Here's how the part is built. I have some questions about the finished solid (model axes, mm). Face numbers are marked on the shaded views. Give positions to 0.01 mm unless a question says otherwise; leave off trailing zeros. Write each loop counter-clockwise with the first axis right and the second up, starting at its lowest first coordinate (ties: lowest second). Pieces come first, ordered by that corner, then holes. Notation, with made-up numbers: (1.25, -22) - (35.25, -22) arc R18 cw to (35.25, 8) - close; hole circle Ø2 at (57, 34.25). An arc over 180 degrees is marked (long way). Use one line per item in the form item = value. Start each with the question number.
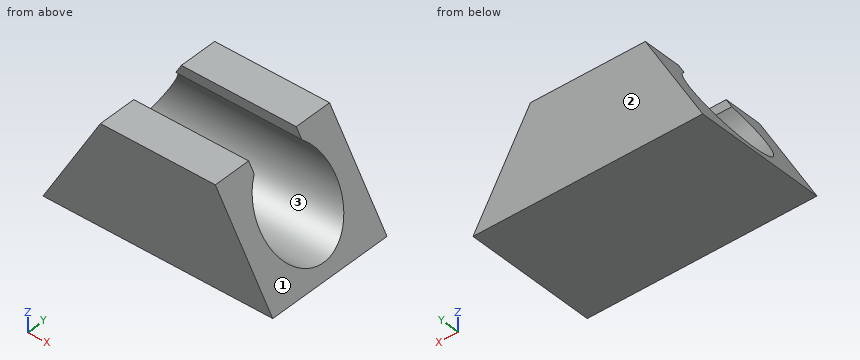
from build123d import *

# Parameters (mm, degrees)
SKETCH8_W           = 10.392304846
SKETCH8_H           = 6
BOSS_EXTRUDE3_DEPTH = 4.5
CUT_EXTRUDE5_DEPTH  = 11.392304845
CUT_EXTRUDE6_DEPTH  = 7


with BuildPart() as part:
    # Sketch8 → Boss-Extrude3 (new body)
    with BuildSketch(Plane.XY):
        Rectangle(SKETCH8_W, SKETCH8_H)
    extrude(amount=BOSS_EXTRUDE3_DEPTH)

    # Sketch9 → Cut-Extrude5 (cut, through all)
    with BuildSketch(Plane(origin=(5.196152423, 0, 0), x_dir=(0, 0, -1), z_dir=(1, 0, 0))):
        with BuildLine():
            Line((-4.0612495, 1.25), (-4.5, 1.25))
            Line((-4.5, 1.25), (-4.5, -1.25))
            Line((-4.5, -1.25), (-4.0612495, -1.25))
            ThreePointArc((-4.0612495, -1.25), (-0.5, 0), (-4.0612495, 1.25))
        make_face()
    extrude(amount=-CUT_EXTRUDE5_DEPTH, mode=Mode.SUBTRACT)

    # Sketch10 → Cut-Extrude6 (cut, through all)
    with BuildSketch(Plane.XZ.offset(3)):
        Polygon((5.196152423, 0), (2.598076211, 4.5), (5.196152423, 4.5), align=None)
        Polygon((-5.196152423, 4.5), (-5.196152423, 0), (-2.598076211, 4.5), align=None)
    extrude(amount=-CUT_EXTRUDE6_DEPTH, mode=Mode.SUBTRACT)


solid = part.part
1. We'd pull the mould along Y, two halves only. Please class the marked faces 1, 2 and 3: pulls with the +Y half, pulls with the -Y half, needs draft (parallel to the pull), parting line crosses it, or undercut.
2. I want a section at C-C, the plane z = 4.25. List the corners of the cut face in (x, y) for me.
3. I want a section at B-B, the plane x = -1.75. List the corners of the cut face in (y, z) for me.
4. I want a section at D-D, the plane y = 2.5. List the corners of the cut face in (x, z) for me, then the cut area to 3 significant figures.
5. I want a section at A-A, the plane z = 1.9. List the corners of the cut face in (x, y) for me.
6. For P1, Ø1.5, axis at y = -2, z = 1, coming from the +X side, with a flat end and sliding along its axis, tell me the tip position at first contact or that it passes through.
7. Please list where these lines run through material, in increasing order: line 1 (Y direction, x = -2, z = 2.5); line 2 (Y direction, x = 2.5, z = 4.2); line 3 (Z direction, x = -3.5, y = 0).
Result sheet:
q1.face_1 = needs draft
q1.face_2 = pulls with the +Y half
q1.face_3 = undercut
q2.outline = (-2.74, -3) - (2.74, -3) - (2.74, -1.25) - (-2.74, -1.25) - close; (-2.74, 1.25) - (2.74, 1.25) - (2.74, 3) - (-2.74, 3) - close
q3.outline = (-3, 0) - (3, 0) - (3, 4.5) - (1.25, 4.5) - (1.25, 4.06) arc R2 cw (long way) to (-1.25, 4.06) - (-1.25, 4.5) - (-3, 4.5) - close
q4.outline = (-5.2, 0) - (5.2, 0) - (2.6, 4.5) - (-2.6, 4.5) - close
q4.area = 35.1 mm2
q5.outline = (-4.1, -3) - (4.1, -3) - (4.1, -1.91) - (-4.1, -1.91) - close; (-4.1, 1.91) - (4.1, 1.91) - (4.1, 3) - (-4.1, 3) - close
q6.P1 = 5.05
q7.line_1 = -3 to -2, 2 to 3
q7.line_2 = -3 to -1.25, 1.25 to 3
q7.line_3 = 0 to 0.5
